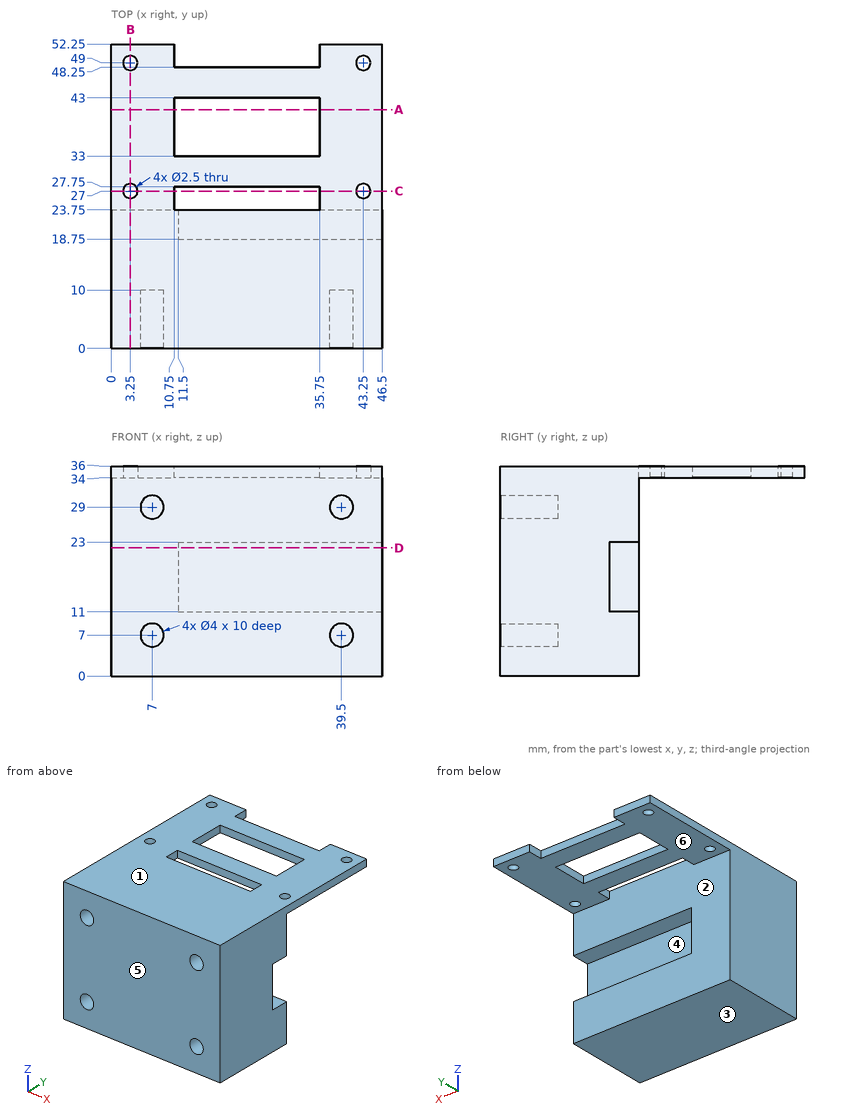
Part print with two shaded views. Sizes in mm from the minimum x, y, z corner. A direction names the side the tool comes from. Coordinates: 2 decimals unless noted, no trailing zeros. Order: outer loops, then holes, each group sorted by start corner. A loop starts at its lowest first (then second) coordinate and runs counter-clockwise, first axis right, second up. Notation, with made-up numbers: (31, 65.5) - (70, 65.5) arc R29 cw to (70, 102.5) - close; hole circle Ø10 at (72.25, 88). An arc over 180 degrees is marked (long way). Write item = value, one per line. Start each with the question number.
1) Saw through at D-D on z = 22. Write the cut outline in (x, y), then the cut area to 3 significant figures.
2) 3-axis set-ups, long thin cutter, end or side, ignore diameter. For the marked faces 5 and 6: which of +Z, -Z, +X, -X, +Y, -Y reach the whole face in a straight line?
3) Two-plate mould, pull along Z, no slides. Class the marked faces 1, 2, 3 and 4: pulls with the +Z half, pulls with the -Z half, needs draft (parallel to the pull), parting line crosses it, or undercut.
4) Saw through at C-C on y = 27. Write the cut outline in (x, z).
5) Wall check: line 1 along Y through (x, z) = (3.25, 35.6); line 2 along X through (y, z) = (5, 7); line 3 along Y through (x, z) = (20, 5). Give the ranges that are in metal, low to high. Write a range as from..to.
6) Saw through at A-A on y = 41. Write the cut outline in (x, z).
7) Saw through at B-B on x = 3.25. Write the cut outline in (y, z), then the cut area to 3 significant figures.
8) Flat gauge pins, fed straight in: pin 1 Ø0.6 at (x, z) = (19, 35.5) entering from +Y; pin 2 Ø1.5 at (x, z) = (29.5, 27.5) entering from -Y; pin 3 Ø2.5 at (y, z) = (22, 15) entering from +X; pin 4 Ø2 at (x, z) = (39.5, 7) entering from -Y. Where does each tip first touch, or does it go through?
From the geometry:
q1.outline = (0, 0) - (46.5, 0) - (46.5, 18.75) - (11.5, 18.75) - (11.5, 23.75) - (0, 23.75) - close
q1.area = 929 mm^2
q2.face_5 = +Z, -Z, +X, -X, -Y
q2.face_6 = -Z, +X, -X, +Y
q3.face_1 = pulls with the +Z half
q3.face_2 = needs draft
q3.face_3 = pulls with the -Z half
q3.face_4 = undercut
q4.outline = (0, 34) - (2, 34) - (2, 36) - (0, 36) - close; (4.5, 34) - (10.75, 34) - (10.75, 36) - (4.5, 36) - close; (35.75, 34) - (42, 34) - (42, 36) - (35.75, 36) - close; (44.5, 34) - (46.5, 34) - (46.5, 36) - (44.5, 36) - close
q5.line_1 = 0..25.75, 28.25..47.75, 50.25..52.25
q5.line_2 = 0..5, 9..37.5, 41.5..46.5
q5.line_3 = 0..23.75
q6.outline = (0, 34) - (10.75, 34) - (10.75, 36) - (0, 36) - close; (35.75, 34) - (46.5, 34) - (46.5, 36) - (35.75, 36) - close
q7.outline = (0, 0) - (23.75, 0) - (23.75, 34) - (25.75, 34) - (25.75, 36) - (0, 36) - close; (28.25, 34) - (47.75, 34) - (47.75, 36) - (28.25, 36) - close; (50.25, 34) - (52.25, 34) - (52.25, 36) - (50.25, 36) - close
q7.area = 902 mm^2
q8.pin_1 = 48.25
q8.pin_2 = 0
q8.pin_3 = 11.5
q8.pin_4 = 10
